For this review, take the finished solid that the model builds, in its own axes (mm). A direction names the side the tool comes from. Round coordinates to 2 decimals unless told otherwise and drop trailing zeros. Order: outer loops, then holes, each group sorted by start corner. A loop starts at its lowest first (then second) coordinate and runs counter-clockwise, first axis right, second up. Notation, with made-up numbers: M -0.75,-1.5 L 37.25,-1.5 A21 cw 37.25,15.5 Z; hole C 1,16 d7. An arc over 180 degrees is marked long. Use a Markdown table: item, result.
from build123d import *

# Parameters (mm, degrees)
F0_R     = 50
F0_R_2   = 44
F1_DEPTH = 30
F2_D     = 30
F3_DEPTH = 210
F4_DEPTH = 85


with BuildPart() as f1:
    # F0 (on Right) → F1 (new body)
    with BuildSketch(Plane.YZ):
        with BuildLine():
            Line((100, -83.066239), (100, 83.066239))
            ThreePointArc((100, 83.066239), (0, 130), (-100, 83.066239))
            Line((-100, 83.066239), (-100, -83.066239))
            ThreePointArc((-100, -83.066239), (0, -130), (100, -83.066239))
        make_face()
        Circle(F0_R, mode=Mode.SUBTRACT)
        Circle(F0_R)
        Circle(F0_R_2, mode=Mode.SUBTRACT)
    extrude(amount=-F1_DEPTH)

    # F2 (through all)
    with Locations(Plane.YZ):
        with Locations((-60, 80), (60, 80), (60, -80), (-60, -80)):
            Hole(F2_D / 2)

    # F0 (on Right) → F3 (join)
    with BuildSketch(Plane.YZ):
        Circle(F0_R)
        Circle(F0_R_2, mode=Mode.SUBTRACT)
    extrude(amount=F3_DEPTH)

    # F0 (on Right) → F4 (join)
    with BuildSketch(Plane.YZ):
        Circle(F0_R)
        Circle(F0_R_2, mode=Mode.SUBTRACT)
    extrude(amount=-F4_DEPTH)


solid = f1.part
Q1. Add section D-D (z = -73). Write out the cut boundary in (x, y).
Determined:
| item | result |
|---|---|
| outline | M -30,-100 L 0,-100 L 0,-73.27 L -30,-73.27 Z; M -30,-46.73 L 0,-46.73 L 0,46.73 L -30,46.73 Z; M -30,73.27 L 0,73.27 L 0,100 L -30,100 Z |
Q2. Draft analysis for pull direction Y (two halves, no side actions). For faces 4 (the cylindrical face through (-15.21, -56.748, -94.643)), 5 (the cylindrical face through (-14.79, -1.6, -129.99)), 6 (the flat face through (-30, 43, 31)), state which applies: pulls with the +Y half, pulls with the -Y half, needs draft (parallel to the pull), parting line crosses it, or undercut.
Determined:
| item | result |
|---|---|
| face 4 | undercut |
| face 5 | parting line crosses it |
| face 6 | needs draft |
Q3. Clearance check with flat-ended pins moving along their axes: pin 1 (5 mm diameter, centred on x = 92.5, y = -46, fed in from +Z); pin 2 (3 mm diameter, centred on x = 136, z = 10, fed in from +Y); pin 3 (1.5 mm diameter, centred on y = -61.5, z = -23, fed in from -X); pin 4 (12 mm diameter, centred on y = -16, z = -39, fed in from +X). State where each tip first meets the part, or that it passes through.
Determined:
| item | result |
|---|---|
| pin 1 | stops at z = 24.65 |
| pin 2 | stops at y = 49.27 |
| pin 3 | stops at x = -30 |
| pin 4 | stops at x = 210 |
Q4. Add section B-B (z = 0). Write out the cut boundary in (x, y), then the cut area to 3 significant figures.
Determined:
| item | result |
|---|---|
| outline | M -85,-50 L -30,-50 L -30,-100 L 0,-100 L 0,-50 L 210,-50 L 210,-44 L -85,-44 Z; M -85,44 L 210,44 L 210,50 L 0,50 L 0,100 L -30,100 L -30,50 L -85,50 Z |
| area | 6,540 mm^2 |
Q5. Wall thickness on line 1 along Z through (x, y) = (77, -1); line 2 along Z through (x, y) = (-11.5, 0); line 3 along Y through (x, z) = (-23, 85.5): over which ranges is each line inside the solid? List them lowest first. Write a range as [from, to].
Determined:
| item | result |
|---|---|
| line 1 | z = [-49.99, -43.99], [43.99, 49.99] |
| line 2 | z = [-130, -44], [44, 130] |
| line 3 | y = [-97.93, -73.96], [-46.04, 46.04], [73.96, 97.93] |
Q6. Add section C-C (y = 65.5). Write out the cut boundary in (x, z), then the cut area to 3 significant figures.
Determined:
| item | result |
|---|---|
| outline | M -30,-112.29 L 0,-112.29 L 0,-93.96 L -30,-93.96 Z; M -30,-66.04 L 0,-66.04 L 0,66.04 L -30,66.04 Z; M -30,93.96 L 0,93.96 L 0,112.29 L -30,112.29 Z |
| area | 5,060 mm^2 |
Q7. Add section A-A (y = 0). Write out the cut boundary in (x, z), then the cut area to 3 significant figures.
Determined:
| item | result |
|---|---|
| outline | M -85,-50 L -30,-50 L -30,-130 L 0,-130 L 0,-50 L 210,-50 L 210,-44 L -85,-44 Z; M -85,44 L 210,44 L 210,50 L 0,50 L 0,130 L -30,130 L -30,50 L -85,50 Z |
| area | 8,340 mm^2 |
Q8. Machinability: for faces 1 (the cylindrical face through (-57.11, 47.69, 15.02)), 2 (the flat face through (0, 43, 31)), 3 (the flat face through (210, -0.2, -44.2)), which of the approach directions +Z, -Z, +X, -X, +Y, -Y give a long, thin tool a straight path to every point of the face, cutting with its end or side? Answer none if there is none.
Determined:
| item | result |
|---|---|
| face 1 | -X |
| face 2 | +X |
| face 3 | +Z, -Z, +X, +Y, -Y |
